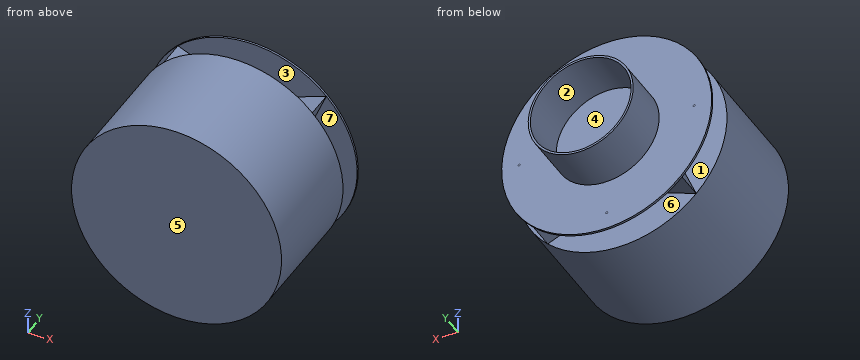
from build123d import *

# Parameters (mm, degrees)
SKETCH11_R          = 304.8
BOSS_EXTRUDE5_DEPTH = 330.2
BOSS_EXTRUDE6_DEPTH = 76.2
SKETCH13_R          = 304.8
BOSS_EXTRUDE7_DEPTH = 6.096
SKETCH14_R          = 152.4
SKETCH14_R_2        = 146.304
BOSS_EXTRUDE8_DEPTH = 139.7
SKETCH16_R          = 3.175
CUT_EXTRUDE2_DEPTH  = 0.0254


with BuildPart() as part:
    # Sketch11 → Boss-Extrude5 (new body)
    with BuildSketch(Plane(origin=(0, 0, 0), x_dir=(1, 0, 0), z_dir=(0, 1, 0))):
        with Locations(Location((0, 0, 0), (0, 0, 270))):
            Circle(SKETCH11_R)
    extrude(amount=BOSS_EXTRUDE5_DEPTH)

    # Sketch12 → Boss-Extrude6 (add)
    with BuildSketch(Plane(origin=(0, 330.2, 0), x_dir=(1, 0, 0), z_dir=(0, 1, 0))):
        Polygon((-127, 0), (-215.526146906, -215.526146906), (0, -127), (215.526146906, -215.526146906), (127, 0), (215.526146906, 215.526146906), (0, 127), (-215.526146906, 215.526146906), align=None)
    extrude(amount=BOSS_EXTRUDE6_DEPTH)

    # Sketch13 → Boss-Extrude7 (add)
    with BuildSketch(Plane(origin=(0, 406.4, 0), x_dir=(1, 0, 0), z_dir=(0, 1, 0))):
        with Locations(Location((0, 0, 0), (0, 0, 135))):
            Circle(SKETCH13_R)
    extrude(amount=BOSS_EXTRUDE7_DEPTH)

    # Sketch14 → Boss-Extrude8 (add)
    with BuildSketch(Plane(origin=(0, 412.496, 0), x_dir=(1, 0, 0), z_dir=(0, 1, 0))):
        with Locations(Location((0, 0, 0), (0, 0, 270))):
            Circle(SKETCH14_R)
        with Locations(Location((0, 0, 0), (0, 0, 270))):
            Circle(SKETCH14_R_2, mode=Mode.SUBTRACT)
    extrude(amount=BOSS_EXTRUDE8_DEPTH)

    # Sketch16 → Cut-Extrude2 (cut)
    with BuildSketch(Plane(origin=(0, 412.496, 0), x_dir=(1, 0, 0), z_dir=(0, 1, 0))):
        with Locations(Location((254, 0, 0), (0, 0, 270))):
            Circle(SKETCH16_R)
        with Locations(Location((0, 254, 0), (0, 0, 270))):
            Circle(SKETCH16_R)
        with Locations(Location((0, -254, 0), (0, 0, 270))):
            Circle(SKETCH16_R)
        with Locations(Location((-254, 0, 0), (0, 0, 270))):
            Circle(SKETCH16_R)
    extrude(amount=-CUT_EXTRUDE2_DEPTH, mode=Mode.SUBTRACT)


solid = part.part
Model file for the job. Use its own axes, mm. Face numbers are marked on the shaded views. A direction names the side the tool comes from. Coordinates: 2 decimals unless noted, no trailing zeros. Write each loop counter-clockwise with the first axis right and the second up, starting at its lowest first coordinate (ties: lowest second). Pieces come first, ordered by that corner, then holes. Notation, with made-up numbers: (-1.75, 38) - (11.25, 38) arc R32 ccw to (11.25, 64) - close; hole circle Ø1 at (19.5, 32.5). An arc over 180 degrees is marked (long way). Write each question's results on one line, items separated by ' | '. Start each with the question number.
1) Probe line 1 along Y through (x, z) = (-274.5, 18.5); line 2 along X through (y, z) = (461.5, -5); line 3 along X through (y, z) = (412.55, 0). List the from-to ranges inside material, lowest first. Write a range as from..to.
2) Flat gauge pins, fed straight in: P1, Ø8, axis at x = 63, y = 192, coming from the +Z side; P2, Ø8, axis at x = 64, y = 464.5, coming from the -Z side; P3, Ø5, axis at x = -254, z = 0, coming from the +Y side. Where does each tip first touch, or does it go through?
3) 3-axis set-ups, long thin cutter, end or side, ignore diameter. For the marked faces 1, 2 and 3: which of +Z, -Z, +X, -X, +Y, -Y reach the whole face in a straight line?
4) Cut at C-C (y = 438). Write the cut outline in (x, z).
5) Cut at A-A (x = -238.5). Write the cut outline in (y, z), then the cut area to 3 significant figures.
6) Cut at D-D (z = -113.5). Write the cut outline in (x, y).
7) Cut at B-B (z = 184). Write the cut outline in (x, y).
8) Mould opens along Y. For the marked faces 4, 5, 6 and 7 say: pulls with the +Y half, pulls with the -Y half, needs draft (parallel to the pull), parting line crosses it, or undercut.
Returned:
1) line 1: 0..330.2, 406.4..412.5 | line 2: -152.32..-146.22, 146.22..152.32 | line 3: -152.4..-146.3, 146.3..152.4
2) P1: z = 299.04 | P2: z = -140.09 | P3: y = 412.47
3) face 1: -X | face 2: +Y | face 3: +Z
4) outline: circle Ø304.8 at (0, 0); hole circle Ø292.61 at (0, 0)
5) outline: (0, -189.79) - (330.2, -189.79) - (330.2, 189.79) - (0, 189.79) - close; (406.4, -189.79) - (412.5, -189.79) - (412.5, 189.79) - (406.4, 189.79) - close | area: 128,000 mm^2
6) outline: (-282.88, 0) - (282.88, 0) - (282.88, 330.2) - (173.62, 330.2) - (173.62, 406.4) - (282.88, 406.4) - (282.88, 412.5) - (101.7, 412.5) - (101.7, 552.2) - (92.32, 552.2) - (92.32, 412.5) - (-92.32, 412.5) - (-92.32, 552.2) - (-101.7, 552.2) - (-101.7, 412.5) - (-282.88, 412.5) - (-282.88, 406.4) - (-173.62, 406.4) - (-173.62, 330.2) - (-282.88, 330.2) - close
7) outline: (-243, 0) - (243, 0) - (243, 330.2) - (202.58, 330.2) - (202.58, 406.4) - (243, 406.4) - (243, 412.5) - (-243, 412.5) - (-243, 406.4) - (-202.58, 406.4) - (-202.58, 330.2) - (-243, 330.2) - close; hole (-138.77, 330.2) - (138.77, 330.2) - (138.77, 406.4) - (-138.77, 406.4) - close
8) face 4: pulls with the +Y half | face 5: pulls with the -Y half | face 6: undercut | face 7: undercut
